Solid Edge part; units mm, degrees
sketch "Sketch1" plane through (0, 0, 0) normal (1, 0, 0) x (0, 1, 0)
  line L0 (-54.4456, 14.5486) -> (45.5544, 14.5486)
  arc A0 (45.5544, -15.4514) -> (45.5544, 14.5486) centre (45.5544, -0.4514) ccw
  line L1 (-54.4456, -15.4514) -> (45.5544, -15.4514)
  arc A1 (-54.4456, 14.5486) -> (-54.4456, -15.4514) centre (-54.4456, -0.4514) ccw
extrude "Protrusion1" add sketch "Sketch1" along normal blind 10
sketch "Sketch2" plane through (0, 0, 0) normal (1, 0, 0) x (0, 1, 0)
  circle A0 centre (-54.4456, -0.4514) radius 4.7659
  circle A1 centre (45.5544, -0.4514) radius 4.7659
extrude "Cutout1" cut sketch "Sketch2" along normal blind 53.975
Design review of the part built by this model. Coordinates are the model's own, in mm. Round coordinates to 2 decimals unless told otherwise and drop trailing zeros. Write each loop counter-clockwise with the first axis right and the second up, starting at its lowest first coordinate (ties: lowest second). Pieces come first, ordered by that corner, then holes.
Item 1: Wall thickness on L1, parallel to Y at x = 0.5, z = -0.25; L2, parallel to Y at x = 8.5, z = -3.75; L3, parallel to Y at x = 7.5, z = -5.25: over which ranges is each line inside the solid? List them lowest first.
Item 2: Consider section D-D on z = -13.5. Give the boundary of the cut face in (x, y).
Item 3: For pin 1 Ø1.5 at (x, z) = (2, 11.5) entering from -Y, flat-tipped, find the tip position at first contact; note if it passes through.
Item 4: Consider section C-C on x = 2. Give the boundary of the cut face in (y, z).
Item 5: Draft analysis for pull direction Z (two halves, no side actions). For faces 1 (the cylindrical face through (4.93, -50.04, 1.37)), 2 (the cylindrical face through (4.93, 60.55, -0.12)), 3 (the flat face through (0, -5, 0)), 4 (the cylindrical face through (4.93, 40.793, -0.661)), state which applies: released by +Z, released by -Z, zero draft, split by the parting line, or undercut.
Item 6: Consider section B-B on z = 2.75. Give the boundary of the cut face in (x, y).
Item 7: Consider section A-A on y = 42.5. Give the boundary of the cut face in (x, z), and give its area (3 significant figures).
Check values:
1. L1: y = -69.44 to -59.21, -49.68 to 40.79, 50.32 to 60.55
1. L2: y = -69.08 to -57.89, -51.01 to 42.11, 48.99 to 60.19
1. L3: y = -68.66 to 59.77
2. outline: (0, -61.84) - (10, -61.84) - (10, 52.95) - (0, 52.95) - close
3. pin 1: stops at y = -64.42
4. outline: (-54.45, -15.45) - (45.55, -15.45) arc R15 ccw to (45.55, 14.55) - (-54.45, 14.55) arc R15 ccw to start; hole circle Ø9.53 at (-54.45, -0.45); hole circle Ø9.53 at (45.55, -0.45)
5. face 1: undercut
5. face 2: split by the parting line
5. face 3: zero draft
5. face 4: undercut
6. outline: (0, -69.1) - (10, -69.1) - (10, -57.98) - (0, -57.98) - close; (0, -50.92) - (10, -50.92) - (10, 42.02) - (0, 42.02) - close; (0, 49.08) - (10, 49.08) - (10, 60.21) - (0, 60.21) - close
7. outline: (0, -15.45) - (10, -15.45) - (10, -4.11) - (0, -4.11) - close; (0, 3.21) - (10, 3.21) - (10, 14.55) - (0, 14.55) - close
7. area: 227 mm2
